Work out the finished part from the listing and answer in its coordinate system (mm). A direction names the side the tool comes from. Give positions to 0.01 mm unless a question says otherwise; leave off trailing zeros. Loops run counter-clockwise (first coordinate to the right, second up) from the corner with the lowest first, then second, coordinate; pieces in that order, holes last. Notation, with made-up numbers: (25, 54) - (77, 54) arc R24 cw to (77, 69) - close; hole circle Ø6 at (63, -35). An arc over 180 degrees is marked (long way). One line per question, with ' | ' between items. Start each with the question number.
1. Which of the six approach directions +Z, -Z, +X, -X, +Y, -Y give full straight-line access (tool end or side, diameter ignored) to faces 4 (the face through (0, 82, 30)), 5 (the face through (65, 10, -45)), 6 (the face through (-1, 52, -60))?
2. Section D-D (x = -48) is taken. Determine the outline of the cut face in (y, z), plus the area to 3 significant figures.
3. Section C-C (y = 12.5) is taken. Determine the outline of the cut face in (x, z).
4. Each of these flat-tipped pins is pushed along its axis until it touches: pin 1 (4.5 mm diameter, centred on y = 79.5, z = -2.5, fed in from -X); pin 2 (8 mm diameter, centred on x = 52, z = 37, fed in from +Y); pin 3 (7.5 mm diameter, centred on y = 37.5, z = -27, fed in from +X). Where does it stop, or does it pass through?
5. Find the intervals of material crossed by line 1 (X direction, y = 7.5, z = -23); line 2 (Y direction, x = -48, z = 62); line 3 (X direction, y = 21.5, z = 70), in increasing order.
6. For a pull along Z with two mould halves and no side action, classify faces 1 (the face through (1, 7, -105)), 2 (the face through (105, 7, 1)), 3 (the face through (31, 14, -49.75)) as released by +Z, released by -Z, zero draft, split by the parting line, or undercut.
Autodesk Inventor part; units mm, degrees
ref_plane "YZ Plane" through (0, 0, 0) normal (1, 0, 0) x (0, 1, 0)
ref_plane "XZ Plane" through (0, 0, 0) normal (0, 1, 0) x (-1, 0, 0)
ref_plane "XY Plane" through (0, 0, 0) normal (0, 0, 1) x (1, 0, 0)
sketch "Náčrt1" plane through (0, 0, 0) normal (0, 1, 0) x (-1, 0, 0)
  line L0 (105, 105) -> (-105, 105)
  line L1 (-105, 105) -> (-105, -105)
  line L2 (-105, -105) -> (105, -105)
  line L3 (105, -105) -> (105, 105)
  line L4 (105, 105) -> (-105, -105) construction
  line L5 (-105, 105) -> (105, -105) construction
  point P0 (0, 0)
  dimension "d0" = 210
  dimension "d1" = 210
extrude "Vysunutí1" add sketch "Náčrt1" along normal blind 15
sketch "Náčrt2" plane through (0, 15, 0) normal (0, 1, 0) x (1, 0, 0)
  line L0 (90, -90) -> (-90, -90)
  line L1 (-90, -90) -> (-90, 90)
  line L2 (-90, 90) -> (90, 90)
  line L3 (90, 90) -> (90, -90)
  line L4 (90, -90) -> (-90, 90) construction
  line L5 (-90, -90) -> (90, 90) construction
  point P0 (0, 0)
  dimension "d4" = 180
  dimension "d5" = 180
extrude "Vysunutí2" add sketch "Náčrt2" along normal blind 15
sketch "Náčrt3" plane through (0, 30, 0) normal (0, 1, 0) x (1, 0, 0)
  line L0 (75, -75) -> (-75, -75)
  line L1 (-75, -75) -> (-75, 75)
  line L2 (-75, 75) -> (75, 75)
  line L3 (75, 75) -> (75, -75)
  line L4 (75, -75) -> (-75, 75) construction
  line L5 (-75, -75) -> (75, 75) construction
  point P0 (0, 0)
  dimension "d8" = 150
  dimension "d9" = 150
extrude "Vysunutí3" add sketch "Náčrt3" along normal blind 15
sketch "Náčrt4" plane through (0, 45, 0) normal (0, 1, 0) x (1, 0, 0)
  line L0 (60, -60) -> (-60, -60)
  line L1 (-60, -60) -> (-60, 60)
  line L2 (-60, 60) -> (60, 60)
  line L3 (60, 60) -> (60, -60)
  line L4 (60, -60) -> (-60, 60) construction
  line L5 (-60, -60) -> (60, 60) construction
  point P0 (0, 0)
  dimension "d12" = 120
  dimension "d13" = 120
extrude "Vysunutí4" add sketch "Náčrt4" along normal blind 15
sketch "Náčrt5" plane through (0, 60, 0) normal (0, 1, 0) x (1, 0, 0)
  line L0 (45, -45) -> (-45, -45)
  line L1 (-45, -45) -> (-45, 45)
  line L2 (-45, 45) -> (45, 45)
  line L3 (45, 45) -> (45, -45)
  line L4 (45, -45) -> (-45, 45) construction
  line L5 (-45, -45) -> (45, 45) construction
  point P0 (0, 0)
  dimension "d16" = 90
  dimension "d17" = 90
extrude "Vysunutí5" add sketch "Náčrt5" along normal blind 15
sketch "Náčrt7" plane through (0, 75, 0) normal (0, 1, 0) x (1, 0, 0)
  line L0 (-30, 30) -> (30, 30)
  line L1 (30, 30) -> (30, -30)
  line L2 (30, -30) -> (-30, -30)
  line L3 (-30, -30) -> (-30, 30)
  line L4 (-30, 30) -> (30, -30) construction
  line L5 (30, 30) -> (-30, -30) construction
  point P0 (0, 0)
  dimension "d20" = 60
  dimension "d21" = 60
extrude "Vysunutí6" add sketch "Náčrt7" along normal blind 15
sketch "Náčrt8" plane through (0, 0, 0) normal (0, -1, 0) x (1, 0, 0)
  line L0 (-55, -55) -> (55, -55)
  line L1 (55, -55) -> (55, 55)
  line L2 (55, 55) -> (-55, 55)
  line L3 (-55, 55) -> (-55, -55)
  line L4 (-55, -55) -> (55, 55) construction
  line L5 (55, -55) -> (-55, 55) construction
  point P0 (0, 0)
  dimension "d24" = 110
  dimension "d25" = 110
extrude "Vysunutí7" cut sketch "Náčrt8" against normal blind 10
sketch "Náčrt9" plane through (0, 0, 0) normal (0, -1, 0) x (1, 0, 0)
  line L0 (55, 55) -> (55, -55)
  line L1 (55, -49.75) -> (65, -49.75)
  line L2 (65, -49.75) -> (65, -39.75)
  line L3 (65, -39.75) -> (55, -39.75)
  line L4 (55, -39.75) -> (55, -49.75)
  line L5 (55, -55) -> (-55, -55)
  point P0 (0, 0)
  dimension "d28" = 10
  dimension "d29" = 10
  dimension "d30" = 5.25
extrude "Vysunutí8" cut sketch "Náčrt9" against normal blind 20
sketch "Náčrt10" plane through (0, 10, 0) normal (0, -1, 0) x (1, 0, 0)
  line L0 (55, -39.75) -> (55, -49.75)
  line L1 (55, -49.75) -> (-2.5, -49.75)
  line L2 (-2.5, -49.75) -> (-2.5, -39.75)
  line L3 (-2.5, -39.75) -> (55, -39.75)
  line L4 (55, -39.75) -> (55, -49.75)
  line L5 (-2.5, -49.75) -> (2.5, -49.75)
  line L6 (2.5, -49.75) -> (2.5, 5)
  line L7 (2.5, 5) -> (-2.5, 5)
  line L8 (-2.5, 5) -> (-2.5, -49.75)
  point P0 (0, 0)
  point P1 (2.5, -39.75)
  dimension "d33" = 57.5
  dimension "d34" = 5
  dimension "d35" = 54.75
extrude "Vysunutí9" cut sketch "Náčrt10" against normal blind 10
properties part number "strecha" material "Dřevo (dub)"
Conclusion:
1) face 4: +Z, +X, -X, +Y | face 5: -Y | face 6: -Z, +X, -X, +Y
2) outline: (0, -105) - (15, -105) - (15, -90) - (30, -90) - (30, -75) - (45, -75) - (45, -60) - (60, -60) - (60, 60) - (45, 60) - (45, 75) - (30, 75) - (30, 90) - (15, 90) - (15, 105) - (0, 105) - (0, 55) - (10, 55) - (10, -55) - (0, -55) - close | area: 8,800 mm²
3) outline: (-105, -105) - (105, -105) - (105, 105) - (-105, 105) - close; hole (-2.5, -49.75) - (65, -49.75) - (65, -39.75) - (2.5, -39.75) - (2.5, 5) - (-2.5, 5) - close
4) pin 1: x = -30 | pin 2: y = 60 | pin 3: x = 75
5) line 1: -105 to -55, 55 to 105 | line 2: 0 to 45 | line 3: -90 to 90
6) face 1: released by -Z | face 2: zero draft | face 3: undercut
